Work out the finished part from the listing and answer in its coordinate system (mm). Face numbers are marked on the shaded views. A direction names the side the tool comes from. Give positions to 0.01 mm unless a question says otherwise; leave off trailing zeros. Order: outer loops, then holes, each group sorted by start corner. A loop starts at its lowest first (then second) coordinate and runs counter-clockwise, first axis right, second up. Notation, with made-up numbers: (40.5, 48) - (82.5, 48) arc R14 ccw to (82.5, 60) - close; hole circle Ø9 at (36.5, 73.5). An arc over 180 degrees is marked (long way). Put each result on its own line as item: value.
```python
from build123d import *

# Parameters (mm, degrees)
F0_W     = 1.8
F0_H     = 1.8
F1_DEPTH = 7.9


with BuildPart() as f1:
    # F0 (on Front) → F1 (new body, symmetric)
    with BuildSketch(Plane.XZ):
        with BuildLine():
            Line((0.9, 0.9), (0.9, 2.3313088598))
            ThreePointArc((0.9, 2.3313088598), (0, 2.499), (-0.9, 2.3313088598))
            Line((-0.9, 2.3313088598), (-0.9, 0.9))
            Line((-0.9, 0.9), (0.9, 0.9))
        make_face()
        with BuildLine():
            Line((2.3313088598, 0.9), (0.9, 0.9))
            Line((0.9, 0.9), (0.9, -0.9))
            Line((0.9, -0.9), (2.3313088598, -0.9))
            ThreePointArc((2.3313088598, -0.9), (2.499, 0), (2.3313088598, 0.9))
        make_face()
        Rectangle(F0_W, F0_H)
        with BuildLine():
            Line((0.9, -2.3313088598), (0.9, -0.9))
            Line((0.9, -0.9), (-0.9, -0.9))
            Line((-0.9, -0.9), (-0.9, -2.3313088598))
            ThreePointArc((-0.9, -2.3313088598), (0, -2.499), (0.9, -2.3313088598))
        make_face()
        with BuildLine():
            Line((-0.9, -0.9), (-0.9, 0.9))
            Line((-0.9, 0.9), (-2.3313088598, 0.9))
            ThreePointArc((-2.3313088598, 0.9), (-2.499, 0), (-2.3313088598, -0.9))
            Line((-2.3313088598, -0.9), (-0.9, -0.9))
        make_face()
    extrude(amount=F1_DEPTH, both=True)


solid = f1.part
```
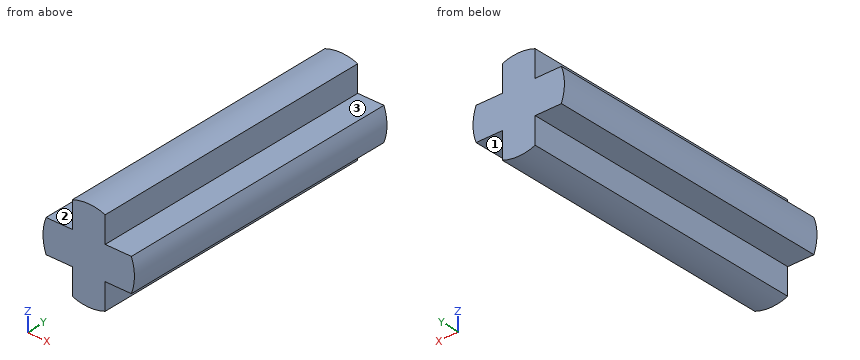
(1) Straight lines are drawn through the part: line 1 (X direction, y = 0.5, z = -2); line 2 (X direction, y = 1.75, z = 0.1). For each, find the intervals that lie inside material, in ascending order.
Geometry check:
line 1: x = -0.9 to 0.9
line 2: x = -2.5 to 2.5
(2) Section C-C, the plane x = -1.8 is taken. Write down the section's boundary in (y, z).
Geometry check:
outline: (-7.9, -0.9) - (7.9, -0.9) - (7.9, 0.9) - (-7.9, 0.9) - close
(3) A tool of negligible diameter and unlimited length cuts with its end or side. For the marked faces 1, 2 and 3, from which of +Z, -Z, +X, -X, +Y, -Y can it reach the whole face along a straight path? Write none if from no direction.
Geometry check:
face 1: -Z, +X, +Y, -Y
face 2: +Z, -X, +Y, -Y
face 3: +Z, +X, +Y, -Y
(4) Section B-B, the plane z = 1.15 is taken. Write down the section's boundary in (x, y).
Geometry check:
outline: (-0.9, -7.9) - (0.9, -7.9) - (0.9, 7.9) - (-0.9, 7.9) - close
(5) Given pin 1 (1.1 mm diameter, centred on x = 1.5, y = 3.5, fed in from -Z); pin 2 (1.6 mm diameter, centred on x = 1.5, y = -1, fed in from +Z); pin 3 (2 mm diameter, centred on y = 6, z = -2, fed in from +X), each flat-ended and moving along its own axis, determine where each tip first touches the part or whether it passes through.
Geometry check:
pin 1: stops at z = -0.9
pin 2: stops at z = 2.4
pin 3: stops at x = 0.9
(6) Section A-A, the plane y = -3.5 is taken. Write down the section's boundary in (x, z), then the cut area to 3 significant figures.
Geometry check:
outline: (-2.33, -0.9) - (-0.9, -0.9) - (-0.9, -2.33) arc R2.5 ccw to (0.9, -2.33) - (0.9, -0.9) - (2.33, -0.9) arc R2.5 ccw to (2.33, 0.9) - (0.9, 0.9) - (0.9, 2.33) arc R2.5 ccw to (-0.9, 2.33) - (-0.9, 0.9) - (-2.33, 0.9) arc R2.5 ccw to start
area: 14.4 mm²
